```python
from build123d import *

# Parameters (mm, degrees)
BOSS_EXTRUDE1_DEPTH    = 6
CUT_EXTRUDE1_DEPTH     = 79.33262411
SKETCH3_W              = 25
SKETCH3_H              = 31.620571099
CUT_EXTRUDE2_DEPTH     = 79.33262411
FILLET1_R              = 3
SKETCH4_R              = 1.75
CUT_EXTRUDE3_DEPTH     = 79.33262411
MOVE_FACE1_OUTLINE_R   = 1.75
MOVE_FACE1_OUTLINE_R_2 = 1.67
MOVE_FACE1_DEPTH       = 6
FILLET2_R              = 1


# Read off the part's stored shape, not the designer's step: Move Face1
with BuildPart() as part:
    # Sketch1 → Boss-Extrude1 (new body)
    with BuildSketch(Plane(origin=(0, 0, 0), x_dir=(1, 0, 0), z_dir=(0, 1, 0))):
        with BuildLine():
            Line((-60, 30), (-60, -30))
            ThreePointArc((-60, -30), (-54.142135624, -44.142135624), (-40, -50))
            Line((-40, -50), (40, -50))
            ThreePointArc((40, -50), (54.142135624, -44.142135624), (60, -30))
            Line((60, -30), (60, 30))
            ThreePointArc((60, 30), (54.142135624, 44.142135624), (40, 50))
            Line((40, 50), (-40, 50))
            ThreePointArc((-40, 50), (-54.142135624, 44.142135624), (-60, 30))
        make_face()
    extrude(amount=BOSS_EXTRUDE1_DEPTH)

    # Sketch2 → Cut-Extrude1 (cut, through all)
    with BuildSketch(Plane(origin=(0, 6, 0), x_dir=(1, 0, 0), z_dir=(0, 1, 0))):
        Polygon((-49, 38), (49, 38), (49, -50), (-46, -50), (-46, -42.5), (-49, -42.5), align=None)
    extrude(amount=-CUT_EXTRUDE1_DEPTH, mode=Mode.SUBTRACT)

    # Sketch3 → Cut-Extrude2 (cut, through all)
    with BuildSketch(Plane(origin=(0, 6, 0), x_dir=(1, 0, 0), z_dir=(0, 1, 0))):
        with Locations((61.5, -32.05028555)):
            Rectangle(SKETCH3_W, SKETCH3_H)
    extrude(amount=-CUT_EXTRUDE2_DEPTH, mode=Mode.SUBTRACT)

    # Fillet1
    fillet1_edges = [part.edges().sort_by_distance(p)[0] for p in [
        (60, 3, 16.24),
    ]]
    fillet(fillet1_edges, radius=FILLET1_R)

    # Sketch4 → Cut-Extrude3 (cut, through all)
    with BuildSketch(Plane(origin=(0, 6, 0), x_dir=(1, 0, 0), z_dir=(0, 1, 0))):
        with Locations(Location((53.475, 0, 0), (0, 0, 270))):
            Circle(SKETCH4_R)
        with Locations(Location((-53.709292606, -36.227375296, 0), (0, 0, 270))):
            Circle(SKETCH4_R)
        with Locations(Location((0, 43.45, 0), (0, 0, 270))):
            Circle(SKETCH4_R)
        with Locations(Location((50.558556763, 40.508556763, 0), (0, 0, 270))):
            Circle(SKETCH4_R)
        with Locations(Location((-50.558556763, 40.508556763, 0), (0, 0, 90))):
            Circle(SKETCH4_R)
    extrude(amount=-CUT_EXTRUDE3_DEPTH, mode=Mode.SUBTRACT)

    # Move Face1 outline → Move Face1 (add)
    # profile 1 of 6: a face of its own
    with BuildSketch(Plane(origin=(0, 0, 0), x_dir=(1, 0, 0), z_dir=(0, 1, 0))):
        with BuildLine():
            ThreePointArc((-40, 50.08), (-54.198704166, 44.198704166), (-60.08, 30))
            Line((-60.08, 30), (-60.08, -30))
            ThreePointArc((-60.08, -30), (-56.156732343, -41.923355232), (-45.92, -49.187495928))
            Line((-45.92, -49.187495928), (-45.92, -42.42))
            Line((-45.92, -42.42), (-48.92, -42.42))
            Line((-48.92, -42.42), (-48.92, 37.92))
            Line((-48.92, 37.92), (48.92, 37.92))
            Line((48.92, 37.92), (48.92, -16.32))
            Line((48.92, -16.32), (57, -16.32))
            ThreePointArc((57, -16.32), (59.177888886, -15.417888886), (60.08, -13.24))
            Line((60.08, -13.24), (60.08, 30))
            ThreePointArc((60.08, 30), (54.198704166, 44.198704166), (40, 50.08))
            Line((40, 50.08), (-40, 50.08))
        make_face()
        with BuildLine():
            Line((-60, -30), (-60, 30))
            ThreePointArc((-60, 30), (-54.142135624, 44.142135624), (-40, 50))
            Line((-40, 50), (40, 50))
            ThreePointArc((40, 50), (54.142135624, 44.142135624), (60, 30))
            Line((60, 30), (60, -13.24))
            ThreePointArc((60, -13.24), (59.121320344, -15.361320344), (57, -16.24))
            Line((57, -16.24), (49, -16.24))
            Line((49, -16.24), (49, 38))
            Line((49, 38), (-49, 38))
            Line((-49, 38), (-49, -42.5))
            Line((-49, -42.5), (-46, -42.5))
            Line((-46, -42.5), (-46, -49.078784028))
            ThreePointArc((-46, -49.078784028), (-56.124515497, -41.832159566), (-60, -30))
        make_face(mode=Mode.SUBTRACT)
    # profile 2 of 6: a face of its own
    with BuildSketch(Plane(origin=(0, 0, 0), x_dir=(1, 0, 0), z_dir=(0, 1, 0))):
        with Locations((53.475, 0)):
            Circle(MOVE_FACE1_OUTLINE_R)
        with Locations((53.475, 0)):
            Circle(MOVE_FACE1_OUTLINE_R_2, mode=Mode.SUBTRACT)
    # profile 3 of 6: a face of its own
    with BuildSketch(Plane(origin=(0, 0, 0), x_dir=(1, 0, 0), z_dir=(0, 1, 0))):
        with Locations((0, 43.45)):
            Circle(MOVE_FACE1_OUTLINE_R)
        with Locations((0, 43.45)):
            Circle(MOVE_FACE1_OUTLINE_R_2, mode=Mode.SUBTRACT)
    # profile 4 of 6: a face of its own
    with BuildSketch(Plane(origin=(0, 0, 0), x_dir=(1, 0, 0), z_dir=(0, 1, 0))):
        with Locations((50.558556763, 40.508556763)):
            Circle(MOVE_FACE1_OUTLINE_R)
        with Locations((50.558556763, 40.508556763)):
            Circle(MOVE_FACE1_OUTLINE_R_2, mode=Mode.SUBTRACT)
    # profile 5 of 6: a face of its own
    with BuildSketch(Plane(origin=(0, 0, 0), x_dir=(1, 0, 0), z_dir=(0, 1, 0))):
        with Locations((-50.558556763, 40.508556763)):
            Circle(MOVE_FACE1_OUTLINE_R)
        with Locations((-50.558556763, 40.508556763)):
            Circle(MOVE_FACE1_OUTLINE_R_2, mode=Mode.SUBTRACT)
    # profile 6 of 6: a face of its own
    with BuildSketch(Plane(origin=(0, 0, 0), x_dir=(1, 0, 0), z_dir=(0, 1, 0))):
        with Locations((-53.709292606, -36.227375296)):
            Circle(MOVE_FACE1_OUTLINE_R)
        with Locations((-53.709292606, -36.227375296)):
            Circle(MOVE_FACE1_OUTLINE_R_2, mode=Mode.SUBTRACT)
    extrude(amount=MOVE_FACE1_DEPTH)

    # Fillet2
    fillet2_edges = [part.edges().sort_by_distance(p)[0] for p in [
        (-45.92, 3, 49.187495928),
    ]]
    fillet(fillet2_edges, radius=FILLET2_R)


solid = part.part
```
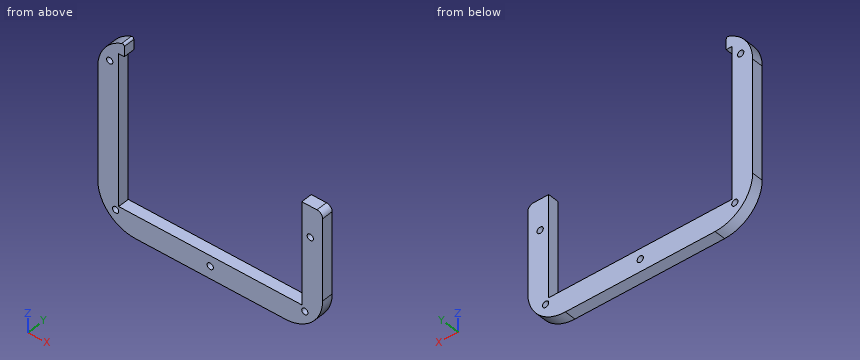
For this review, take the finished solid that the model builds, in its own axes (mm). Coordinates: 2 decimals unless noted, no trailing zeros. Write each loop counter-clockwise with the first axis right and the second up, starting at its lowest first coordinate (ties: lowest second). Pieces come first, ordered by that corner, then holes. Notation, with made-up numbers: (65, -28) - (123, -28) arc R27 cw to (123, 10) - close; hole circle Ø6 at (23.25, 85.5). An arc over 180 degrees is marked (long way). Answer in a Markdown table with one row per item. Add a question column.
Q1. We need section D-D, the plane y = 2.8. State the section outline as (x, z) points (3 decimals).
Q2. For P1, Ø1.8, axis at x = 53, y = 4, coming from the +Z side; P2, Ø3, axis at x = -13.5, y = 2.5, coming from the +Z side; P3, Ø1.6, axis at y = 3, z = 44, coming from the +X side, all flat-tipped, find the tip position at first contact; note any pin that passes through.
Q3. For probe 1 along X at (y, z) = (1.3, 0) (3 decimals); probe 2 along X at (y, z) = (1.9, -25); probe 3 along X at (y, z) = (5.25, -42), list the stretches that pass through material, from the lowest coordinate up.
Q4. We need section A-A, the plane z = -11.5. State the section outline as (x, y) points, and give its area (3 significant figures).
Q5. We need section B-B, the plane x = 0. State the section outline as (y, z) points.
Q6. We need section C-C, the plane z = 0. State the section outline as (x, y) points (3 decimals).
Answer list:
| question | item | result |
|---|---|---|
| 1 | outline | (-60.08, -30) arc R20.08 ccw to (-40, -50.08) - (40, -50.08) arc R20.08 ccw to (60.08, -30) - (60.08, 13.24) arc R3.08 ccw to (57, 16.32) - (48.92, 16.32) - (48.92, -37.92) - (-48.92, -37.92) - (-48.92, 42.42) - (-45.92, 42.42) - (-45.92, 47.781) arc R1 ccw to (-47.283, 48.713) arc R20.08 ccw to (-60.08, 30) - close; hole circle Ø3.34 at (-53.709, 36.227); hole circle Ø3.34 at (-50.559, -40.509); hole circle Ø3.34 at (0, -43.45); hole circle Ø3.34 at (50.559, -40.509); hole circle Ø3.34 at (53.475, 0) |
| 2 | P1 | stops at z = 16.32 |
| 2 | P2 | stops at z = -37.92 |
| 2 | P3 | stops at x = -45.92 |
| 3 | probe 1 | x = -60.08 to -48.92, 48.92 to 51.805, 55.145 to 60.08 |
| 3 | probe 2 | x = -60.08 to -48.92, 48.92 to 60.08 |
| 3 | probe 3 | x = -56.1 to -51.31, -49.81 to -0.83, 0.83 to 49.81, 51.31 to 56.1 |
| 4 | outline | (-60.08, 0) - (-48.92, 0) - (-48.92, 6) - (-60.08, 6) - close; (48.92, 0) - (60.08, 0) - (60.08, 6) - (48.92, 6) - close |
| 4 | area | 134 mm2 |
| 5 | outline | (0, -50.08) - (6, -50.08) - (6, -45.12) - (0, -45.12) - close; (0, -41.78) - (6, -41.78) - (6, -37.92) - (0, -37.92) - close |
| 6 | outline | (-60.08, 0) - (-48.92, 0) - (-48.92, 6) - (-60.08, 6) - close; (48.92, 0) - (51.805, 0) - (51.805, 6) - (48.92, 6) - close; (55.145, 0) - (60.08, 0) - (60.08, 6) - (55.145, 6) - close |
